from build123d import *

# Parameters (mm, degrees)
SKETCH_R              = 26
PAD_DEPTH             = 15
SKETCH001_R           = 2.25
POCKET_DEPTH          = 16
POLARPATTERN_COUNT    = 3
SKETCH002_R           = 2.75
POCKET001_DEPTH       = 15
POLARPATTERN001_COUNT = 3


with BuildPart() as part:
    # Sketch → Pad (new body)
    with BuildSketch(Plane.XY):
        with BuildLine():
            Line((-22.5, 30), (22.5, 30))
            ThreePointArc((37.2307621135, 4.4855715852), (32.4759535891, 18.7500005468), (22.5, 30))
            Line((37.2307621135, 4.4855715852), (14.7307621135, -34.4855715852))
            ThreePointArc((-14.7307621135, -34.4855715852), (0, -37.5000010954), (14.7307621135, -34.4855715852))
            Line((-14.7307621135, -34.4855715852), (-37.2307621135, 4.4855715851))
            ThreePointArc((-22.5, 30), (-32.475953589, 18.7500005468), (-37.2307621135, 4.4855715852))
        make_face()
        Circle(SKETCH_R, mode=Mode.SUBTRACT)
    extrude(amount=PAD_DEPTH)

    # Sketch001 (on DatumPlane) → Pocket (cut)
    with BuildSketch(Plane(origin=(25.9807621135, -15, 0), x_dir=(0.5, 0.8660254038, 0), z_dir=(0.8660254038, -0.5, 0))):
        with Locations((-17.5, 7.5)):
            Circle(SKETCH001_R)
        with Locations((17.5, 7.5)):
            Circle(SKETCH001_R)
    pocket = extrude(amount=-POCKET_DEPTH, mode=Mode.SUBTRACT)

    # PolarPattern: Pocket ×3 about axis
    polarpattern_axis = Axis((0, 0, 0), (0, 0, 1))
    for i in range(1, POLARPATTERN_COUNT):
        add(pocket.rotate(polarpattern_axis, i * 360 / POLARPATTERN_COUNT), mode=Mode.SUBTRACT)

    # Sketch002 (on DatumPlane) → Pocket001 (cut, symmetric)
    with BuildSketch(Plane(origin=(-31.6010078868, 18.2448504101, 7.5), x_dir=(0, 0, 1), z_dir=(0.8660254038, -0.5, 0))):
        Circle(SKETCH002_R)
    pocket001 = extrude(amount=POCKET001_DEPTH, both=True, mode=Mode.SUBTRACT)

    # PolarPattern001: Pocket001 ×3 about axis
    polarpattern001_axis = Axis((0, 0, 0), (0, 0, 1))
    for i in range(1, POLARPATTERN001_COUNT):
        add(pocket001.rotate(polarpattern001_axis, i * 360 / POLARPATTERN001_COUNT), mode=Mode.SUBTRACT)


solid = part.part
Input: part model. Units: mm. Frame: model coordinates. A direction names the side the tool comes from. Coordinates: 2 decimals unless noted, no trailing zeros. Order: outer loops, then holes, each group sorted by start corner. A loop starts at its lowest first (then second) coordinate and runs counter-clockwise, first axis right, second up.
1. Contact query for flat-ended pins moving along their axis: P1, Ø6, axis at y = 5.5, z = 2, coming from the -X side; P2, Ø3, axis at x = -24.5, z = 2, coming from the -Y side; P3, Ø1.5, axis at y = 0, z = 11.5, coming from the +X side; P4, Ø3.5, axis at x = 0, z = 7.5, coming from the -Y side. Output: stop coordinate, or through.
Checked values:
P1: stops at x = -37.23
P2: stops at y = -20.16
P3: stops at x = 35.07
P4: stops at y = 25.94
2. Cut plane A-A, the plane x = 0. Return loops of the section in (y, z).
Checked values:
outline: (-37.5, 0) - (-26, 0) - (-26, 4.75) - (-37.5, 4.75) - close; (-37.5, 10.25) - (-26, 10.25) - (-26, 15) - (-37.5, 15) - close; (26, 0) - (30, 0) - (30, 15) - (26, 15) - close
3. Ray query, line 1 along Z through (x, y) = (0, -32); line 2 along Z through (x, y) = (17.5, 20.5); line 3 along Y through (x, z) = (-0.5, 12). Return the intervals inside material, ascending.
Checked values:
line 1: z = 0 to 4.75, 10.25 to 15
line 2: z = 0 to 5.25, 9.75 to 15
line 3: y = -37.5 to -26, 26 to 30
4. Cut plane C-C, the plane z = 7.5. Count the separate pieces of the cut face and the enclosed holes in it, plus the area to 3 significant figures.
Checked values:
separate pieces: 9
enclosed holes: 0
area: 1,120 mm2
5. Cut plane B-B, the plane z = 3.25. Return loops of the section in (x, y), plus the area to 3 significant figures.
Checked values:
outline: (-37.23, 4.49) - (-14.73, -34.49) arc R37.5 ccw to (14.73, -34.49) - (37.23, 4.49) arc R37.5 ccw to (22.5, 30) - (-22.5, 30) arc R37.5 ccw to start; hole circle Ø52 at (0, 0)
area: 1,600 mm2
6. Access query for faces 5 (the cylindrical face through (-3.57, -37.33, 7.4)), 6 (the cylindrical face through (-19.646, 25.001, 8.176)), 7 (the cylindrical face through (0.83, -31.6, 10.12)). Directions: +Z, -Z, +X, -X, +Y, -Y. A direction counts if a zero-diameter tool reaches every point of the face in a straight line with its end or side. Return the directions, or none.
Checked values:
face 5: +Z, -Z, -Y
face 6: +Y
face 7: -Y
7. Draft query along Z for faces 1 (the flat face through (-3, -26, 0)), 2 (the flat face through (-3, -26, 15)), 3 (the flat face through (0, 30, 7)), 4 (the cylindrical face through (-11.828, -29.514, 8.176)). Return one class per face: +Z half, -Z half, draft (parallel to the pull), parting line (faces both ways), or undercut.
Checked values:
face 1: -Z half
face 2: +Z half
face 3: draft
face 4: undercut
